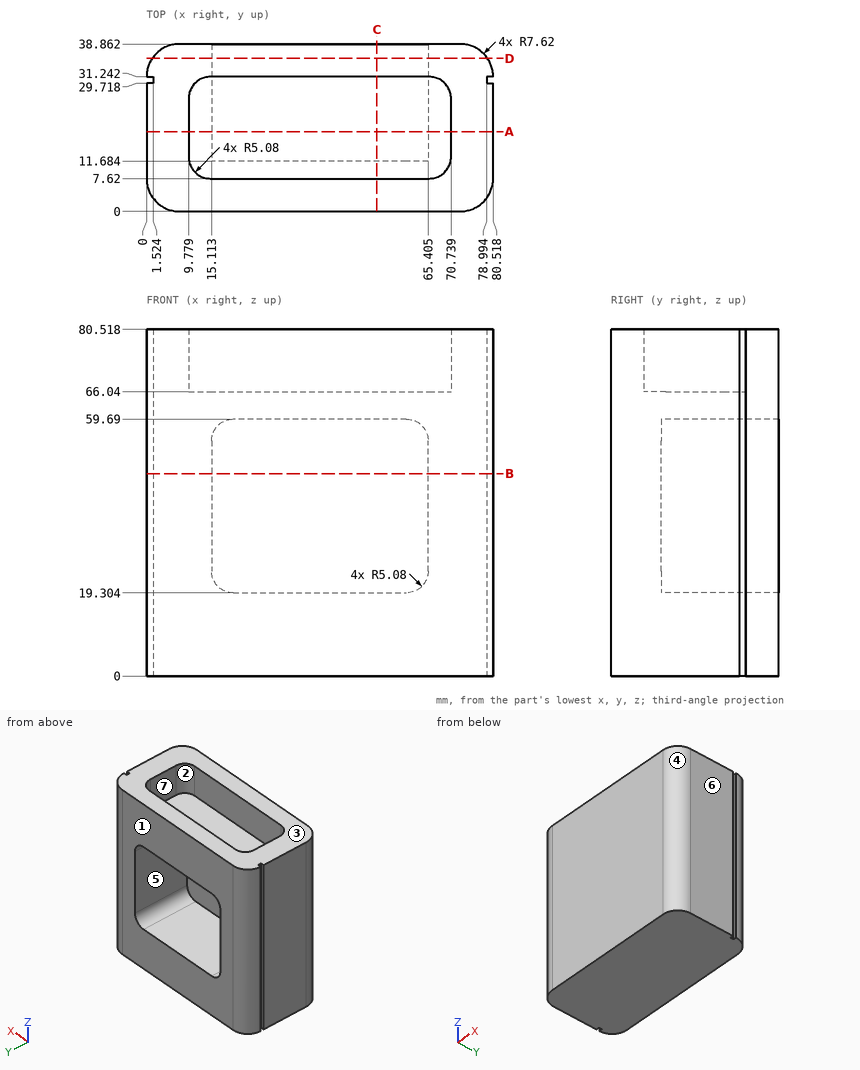
Print and shaded views of the part. All mm, measured from the part's lowest x, y and z. A direction names the side the tool comes from. Round coordinates to 2 decimals unless told otherwise and drop trailing zeros. Write each loop counter-clockwise with the first axis right and the second up, starting at its lowest first coordinate (ties: lowest second). Pieces come first, ordered by that corner, then holes. Notation, with made-up numbers: (16.5, -8) -> (49.5, -8) arc R36 ccw to (49.5, 26) -> close; hole circle Ø10 at (-17.5, 55.5). An arc over 180 degrees is marked (long way). Answer in a Markdown table with one row per item. Add a question column.
Item 1: Drop flat-ended pins along their axis: pin 1 Ø0.5 at (x, z) = (1, 37) entering from +Y; pin 2 Ø6 at (y, z) = (34.5, 29) entering from +X; pin 3 Ø8 at (x, y) = (30.5, 25) entering from +Z. Give the stop position or say it passes through.
Item 2: Drill centre lines: line 1 (X direction, y = 31, z = 41) (3 decimals); line 2 (Y direction, x = 66, z = 73); line 3 (X direction, y = 16, z = 39.5) (3 decimals). Where is each one in solid material? Low to high. Write a range as from..to.
Item 3: Saw through at B-B, the plane z = 47. Write the cut outline in (x, y) (3 decimals).
Item 4: Saw through at D-D, the plane y = 35.5. Write the cut outline in (x, z) (3 decimals).
Item 5: Mould opens along Y. For the marked faces 1, 2, 3 and 4 say: pulls with the +Y half, pulls with the -Y half, needs draft (parallel to the pull), parting line crosses it, or undercut.
Item 6: Which spindle directions (+Z, -Z, +X, -X, +Y, -Y) get a long thin tool onto all of the face, cutting with end or side? Do the marked faces 5, 6 and 7. Say none if no direction does.
Item 7: Saw through at C-C, the plane x = 53.5. Write the cut outline in (y, z), then the cut area to 3 significant figures.
Item 8: Saw through at A-A, the plane y = 18.5. Write the cut outline in (x, z) (3 decimals).
Findings below:
| question | item | result |
|---|---|---|
| 1 | pin 1 | stops at y = 35.42 |
| 1 | pin 2 | stops at x = 80.51 |
| 1 | pin 3 | stops at z = 66.04 |
| 2 | line 1 | x = 1.524..15.113, 65.405..78.994 |
| 2 | line 2 | y = 0..7.63, 31.23..38.86 |
| 2 | line 3 | x = 0..15.113, 65.405..80.518 |
| 3 | outline | (0, 7.62) arc R7.62 ccw to (7.62, 0) -> (72.898, 0) arc R7.62 ccw to (80.518, 7.62) -> (80.518, 29.718) -> (78.994, 29.718) -> (78.994, 31.242) -> (80.518, 31.242) arc R7.62 ccw to (72.898, 38.862) -> (65.405, 38.862) -> (65.405, 11.684) -> (15.113, 11.684) -> (15.113, 38.862) -> (7.62, 38.862) arc R7.62 ccw to (0, 31.242) -> (1.524, 31.242) -> (1.524, 29.718) -> (0, 29.718) -> close |
| 4 | outline | (1.301, 0) -> (79.217, 0) -> (79.217, 80.518) -> (1.301, 80.518) -> close; hole (15.113, 24.384) arc R5.08 ccw to (20.193, 19.304) -> (60.325, 19.304) arc R5.08 ccw to (65.405, 24.384) -> (65.405, 54.61) arc R5.08 ccw to (60.325, 59.69) -> (20.193, 59.69) arc R5.08 ccw to (15.113, 54.61) -> close |
| 5 | face 1 | pulls with the +Y half |
| 5 | face 2 | undercut |
| 5 | face 3 | needs draft |
| 5 | face 4 | pulls with the -Y half |
| 6 | face 5 | +Y |
| 6 | face 6 | +Z, -Z, +X, +Y, -Y |
| 6 | face 7 | +Z |
| 7 | outline | (0, 0) -> (38.86, 0) -> (38.86, 19.3) -> (11.68, 19.3) -> (11.68, 59.69) -> (38.86, 59.69) -> (38.86, 80.52) -> (31.24, 80.52) -> (31.24, 66.04) -> (7.62, 66.04) -> (7.62, 80.52) -> (0, 80.52) -> close |
| 7 | area | 1,690 mm^2 |
| 8 | outline | (0, 0) -> (80.518, 0) -> (80.518, 80.518) -> (70.739, 80.518) -> (70.739, 66.04) -> (9.779, 66.04) -> (9.779, 80.518) -> (0, 80.518) -> close; hole (15.113, 24.384) arc R5.08 ccw to (20.193, 19.304) -> (60.325, 19.304) arc R5.08 ccw to (65.405, 24.384) -> (65.405, 54.61) arc R5.08 ccw to (60.325, 59.69) -> (20.193, 59.69) arc R5.08 ccw to (15.113, 54.61) -> close |
